For this review, take the finished solid that the model builds, in its own axes (mm). A direction names the side the tool comes from. Coordinates: 2 decimals unless noted, no trailing zeros. Write each loop counter-clockwise with the first axis right and the second up, starting at its lowest first coordinate (ties: lowest second). Pieces come first, ordered by that corner, then holes.
1) For faces 4 (the face through (20, -11, -59)), 5 (the face through (0, -7.685, -59)), 6 (the face through (-8.113, -11.006, -59.16)), list the 3-axis set-ups (+Z, -Z, +X, -X, +Y, -Y) from which the entire face can be reached by the end or side of a thin tool; tool diameter is ignored.
2) Insertion check: P1, Ø3, axis at y = -1.5, z = -48, coming from the -X side; P2, Ø0.9, axis at x = -17.5, z = -46, coming from the -Y side; P3, Ø1.1, axis at y = 18, z = -80, coming from the +X side. Each pin has a flat end and moves straight along its axis. Give the tip position at first contact, or say it passes through.
3) Mouldability with a two-part tool opening along X and no side actions: class faces 1 (the face through (-11, -20, -59)), 2 (the face through (7.685, 0, -59)), 3 (the face through (0, 7.685, -59)) as pulls with the +X half, pulls with the -X half, needs draft (parallel to the pull), parting line crosses it, or undercut.
4) To check wall thickness, follow line 1 along Y through (x, z) = (0, -79) (3 decimals); line 2 along Y through (x, z) = (5, -68); line 3 along X through (y, z) = (14, -70). State the ranges of each line that lie inside material, in increasing order.
5) We need section A-A on y = 0. Write out the cut boundary in (x, z) (3 decimals), then the cut area to 3 significant figures.
from build123d import *

# Parameters (mm, degrees)
SKETCH1_R      = 3.4
EXTRUDE1_DEPTH = 120


with BuildPart() as part:
    # Sketch1 → Extrude1 (new body)
    with BuildSketch(Plane.XY):
        with BuildLine():
            Line((-8.715, -15.524615034), (-5.63, -15.524615034))
            ThreePointArc((-5.63, -15.524615034), (-4.519842354, -15.984457388), (-4.06, -17.094615034))
            Line((-4.06, -17.094615034), (-4.06, -18.43))
            ThreePointArc((-4.06, -18.43), (-4.519842354, -19.540157646), (-5.63, -20))
            Line((-5.63, -20), (-16.674615034, -20))
            ThreePointArc((-16.674615034, -20), (-18.951578385, -19.194274381), (-20, -17.018368134))
            Line((-20, -17.018368134), (-20, -5.757918808))
            ThreePointArc((-20, -5.757918808), (-19.564709668, -4.603883664), (-18.43, -4.120449326))
            Line((-18.43, -4.120449326), (-17.25, -4.120449326))
            ThreePointArc((-17.25, -4.120449326), (-16.115287682, -4.60388249), (-15.67999625, -5.757919334))
            Line((-15.67999625, -5.757919334), (-15.67999625, -8.715399492))
            ThreePointArc((-15.67999625, -8.715399492), (-15.220153896, -9.825557139), (-14.10999625, -10.285399492))
            Line((-14.10999625, -10.285399492), (-13.816898819, -10.285399492))
            ThreePointArc((-13.816898819, -10.285399492), (-13.526061711, -10.227547119), (-13.279501941, -10.062800646))
            Line((-13.279501941, -10.062800646), (-9.076242789, -5.859541495))
            ThreePointArc((-9.076242789, -5.859541495), (-8.046572221, -4.318530588), (-7.685, -2.500784284))
            Line((-7.685, -2.500784284), (-7.685, 2.500784284))
            ThreePointArc((-7.685, 2.500784284), (-8.046572221, 4.318530588), (-9.076242789, 5.859541495))
            Line((-9.076242789, 5.859541495), (-13.040489136, 9.823787841))
            ThreePointArc((-13.040489136, 9.823787841), (-13.354224618, 10.012729352), (-13.71989919, 10.033001362))
            Line((-13.71989919, 10.033001362), (-14.05520779, 10.044710596))
            ThreePointArc((-14.05520779, 10.044710596), (-15.200613642, 9.605030484), (-15.68, 8.475666998))
            Line((-15.68, 8.475666998), (-15.68, 5.572979049))
            ThreePointArc((-15.68, 5.572979049), (-16.139842354, 4.462821403), (-17.25, 4.002979049))
            Line((-17.25, 4.002979049), (-18.43, 4.002979049))
            ThreePointArc((-18.43, 4.002979049), (-19.540157646, 4.462821403), (-20, 5.572979049))
            Line((-20, 5.572979049), (-20, 13.004526564))
            Line((-20, 13.004526564), (-20, 16.83))
            ThreePointArc((-20, 16.83), (-19.071528496, 19.071528496), (-16.83, 20))
            Line((-16.83, 20), (-5.63, 20))
            ThreePointArc((-5.63, 20), (-4.519842354, 19.540157646), (-4.06, 18.43))
            Line((-4.06, 18.43), (-4.06, 17.094615034))
            ThreePointArc((-4.06, 17.094615034), (-4.519842354, 15.984457388), (-5.63, 15.524615034))
            Line((-5.63, 15.524615034), (-8.715, 15.524615034))
            ThreePointArc((-8.715, 15.524615034), (-9.825157646, 15.06477268), (-10.285, 13.954615034))
            Line((-10.285, 13.954615034), (-10.285, 13.492503602))
            ThreePointArc((-10.285, 13.492503602), (-10.227148445, 13.201664194), (-10.062401154, 12.955102448))
            Line((-10.062401154, 12.955102448), (-6.217092793, 9.109794088))
            ThreePointArc((-6.217092793, 9.109794088), (-4.63891877, 8.055291919), (-2.777335583, 7.685))
            Line((-2.777335583, 7.685), (2.777335583, 7.685))
            ThreePointArc((2.777335583, 7.685), (4.63891877, 8.055291919), (6.217092793, 9.109794088))
            Line((6.217092793, 9.109794088), (10.062401154, 12.955102448))
            ThreePointArc((10.062401154, 12.955102448), (10.227148445, 13.201664194), (10.285, 13.492503602))
            Line((10.285, 13.492503602), (10.285, 13.954615034))
            ThreePointArc((10.285, 13.954615034), (9.825157646, 15.06477268), (8.715, 15.524615034))
            Line((8.715, 15.524615034), (5.63, 15.524615034))
            ThreePointArc((5.63, 15.524615034), (4.519842354, 15.984457388), (4.06, 17.094615034))
            Line((4.06, 17.094615034), (4.06, 18.43))
            ThreePointArc((4.06, 18.43), (4.519842354, 19.540157646), (5.63, 20))
            Line((5.63, 20), (12.979635074, 20))
            Line((12.979635074, 20), (16.83, 20))
            ThreePointArc((16.83, 20), (19.071528496, 19.071528496), (20, 16.83))
            Line((20, 16.83), (20, 13.001098436))
            Line((20, 13.001098436), (20, 5.63))
            ThreePointArc((20, 5.63), (19.540157461, 4.519842693), (18.43, 4.060000526))
            Line((18.43, 4.060000526), (17.24999625, 4.060000526))
            ThreePointArc((17.24999625, 4.060000526), (16.139838603, 4.519842879), (15.67999625, 5.630000526))
            Line((15.67999625, 5.630000526), (15.67999625, 8.715399492))
            ThreePointArc((15.67999625, 8.715399492), (15.220153896, 9.825557139), (14.10999625, 10.285399492))
            Line((14.10999625, 10.285399492), (13.816903094, 10.285399492))
            ThreePointArc((13.816903094, 10.285399492), (13.526063686, 10.227547937), (13.279501941, 10.062800646))
            Line((13.279501941, 10.062800646), (9.076242789, 5.859541495))
            ThreePointArc((9.076242789, 5.859541495), (8.046572221, 4.318530588), (7.685, 2.500784284))
            Line((7.685, 2.500784284), (7.685, -2.500784284))
            ThreePointArc((7.685, -2.500784284), (8.046572221, -4.318530588), (9.076242789, -5.859541495))
            Line((9.076242789, -5.859541495), (13.163657296, -9.946956002))
            ThreePointArc((13.163657296, -9.946956002), (13.35903797, -10.160433474), (13.6200547, -10.285399492))
            Line((13.6200547, -10.285399492), (14.10999625, -10.285399492))
            ThreePointArc((14.10999625, -10.285399492), (15.220153896, -9.825557139), (15.67999625, -8.715399492))
            Line((15.67999625, -8.715399492), (15.67999625, -5.630000526))
            ThreePointArc((15.67999625, -5.630000526), (16.139838603, -4.519842879), (17.24999625, -4.060000526))
            Line((17.24999625, -4.060000526), (18.43, -4.060000526))
            ThreePointArc((18.43, -4.060000526), (19.540157461, -4.519842693), (20, -5.63))
            Line((20, -5.63), (20, -16.83))
            ThreePointArc((20, -16.83), (19.071528496, -19.071528496), (16.83, -20))
            Line((16.83, -20), (13, -20))
            Line((13, -20), (5.63, -20))
            ThreePointArc((5.63, -20), (4.519842354, -19.540157646), (4.06, -18.43))
            Line((4.06, -18.43), (4.06, -17.094615034))
            ThreePointArc((4.06, -17.094615034), (4.519842354, -15.984457388), (5.63, -15.524615034))
            Line((5.63, -15.524615034), (8.715, -15.524615034))
            ThreePointArc((8.715, -15.524615034), (9.825157646, -15.06477268), (10.285, -13.954615034))
            Line((10.285, -13.954615034), (10.285, -13.492503602))
            ThreePointArc((10.285, -13.492503602), (10.227148445, -13.201664194), (10.062401154, -12.955102448))
            Line((10.062401154, -12.955102448), (6.217092793, -9.109794088))
            ThreePointArc((6.217092793, -9.109794088), (4.63891877, -8.055291919), (2.777335583, -7.685))
            Line((2.777335583, -7.685), (-2.777335583, -7.685))
            ThreePointArc((-2.777335583, -7.685), (-4.63891877, -8.055291919), (-6.217092793, -9.109794088))
            Line((-6.217092793, -9.109794088), (-10.062401154, -12.955102448))
            ThreePointArc((-10.062401154, -12.955102448), (-10.227148445, -13.201664194), (-10.285, -13.492503602))
            Line((-10.285, -13.492503602), (-10.285, -13.954615034))
            ThreePointArc((-10.285, -13.954615034), (-9.825157646, -15.06477268), (-8.715, -15.524615034))
        make_face()
        Circle(SKETCH1_R, mode=Mode.SUBTRACT)
    extrude(amount=-EXTRUDE1_DEPTH)


solid = part.part
Result:
1. face 4: +Z, -Z, +X, +Y, -Y
1. face 5: +Z, -Z, -Y
1. face 6: +Z, -Z
2. P1: stops at x = -7.71
2. P2: stops at y = -20
2. P3: stops at x = 19.94
3. face 1: needs draft
3. face 2: pulls with the +X half
3. face 3: undercut
4. line 1: y = -7.685 to -3.4, 3.4 to 7.685
4. line 2: y = -19.87 to -15.66, -8.22 to 8.22, 15.66 to 19.87
4. line 3: x = -20 to -10.28, 10.28 to 20
5. outline: (-7.685, -120) - (-3.4, -120) - (-3.4, 0) - (-7.685, 0) - close; (3.4, -120) - (7.685, -120) - (7.685, 0) - (3.4, 0) - close
5. area: 1,030 mm2
